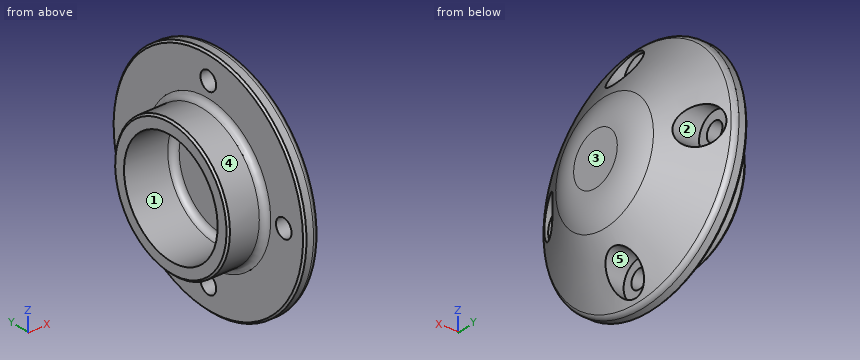
```python
from build123d import *

# Parameters (mm, degrees)
FILLET2_R          = 1
CHAMFER1_SIZE      = 0.3
SKETCH2_R          = 1.5
CUT_EXTRUDE1_DEPTH = 10
SKETCH3_R          = 3
CUT_EXTRUDE2_DEPTH = 10


with BuildPart() as part:
    # Sketch1 → Revolve1 (revolve)
    with BuildSketch(Plane.XY, mode=Mode.PRIVATE) as revolve1_sk:
        with BuildLine():
            Line((-6, 9), (-6, 11))
            Line((-6, 11), (0, 11))
            Line((0, 11), (0, 18.5))
            Line((0, 18.5), (1.438007651, 18.5))
            ThreePointArc((1.438007651, 18.5), (1.927932672, 18.371764575), (2.292206206, 18.019946947))
            Line((2.292206206, 18.019946947), (7.541985556, 9.395309443))
            ThreePointArc((7.541985556, 9.395309443), (8.628599471, 6.895853348), (9, 4.195839975))
            Line((9, 4.195839975), (9, 0))
            Line((9, 0), (2, 0))
            Line((2, 0), (2, 9))
            Line((2, 9), (-6, 9))
        make_face()
    revolve(revolve1_sk.sketch.rotate(Axis((0, 0, 0), (1, 0, 0)), 90), axis=Axis((0, 0, 0), (1, 0, 0)))

    # Fillet2
    fillet2_edges = [part.edges().sort_by_distance(p)[0] for p in [
        (0, 0, -11),
        (2, 0, -9),
    ]]
    fillet(fillet2_edges, radius=FILLET2_R)

    # Chamfer1
    chamfer1_edges = [part.edges().sort_by_distance(p)[0] for p in [
        (0, 0, -18.5),
        (-6, 0, -11),
    ]]
    chamfer(chamfer1_edges, length=CHAMFER1_SIZE)

    # Sketch2 → Cut-Extrude1 (cut)
    with BuildSketch(Plane.ZY):
        with Locations((0, 14.5)):
            Circle(SKETCH2_R)
        with Locations((14.5, 0)):
            Circle(SKETCH2_R)
        with Locations((0, -14.5)):
            Circle(SKETCH2_R)
        with Locations((-14.5, 0)):
            Circle(SKETCH2_R)
    extrude(amount=-CUT_EXTRUDE1_DEPTH, mode=Mode.SUBTRACT)

    # Sketch3 → Cut-Extrude2 (cut)
    with BuildSketch(Plane.ZY.offset(-2)):
        with Locations((0, 14.5)):
            Circle(SKETCH3_R)
        with Locations((14.5, 0)):
            Circle(SKETCH3_R)
        with Locations((0, -14.5)):
            Circle(SKETCH3_R)
        with Locations((-14.5, 0)):
            Circle(SKETCH3_R)
    extrude(amount=-CUT_EXTRUDE2_DEPTH, mode=Mode.SUBTRACT)


solid = part.part
```
Read the model definition and answer for the solid it produces. Units are mm, in the model's axes. Face numbers are marked on the shaded views. A direction names the side the tool comes from. Round coordinates to 2 decimals unless told otherwise and drop trailing zeros. Write each loop counter-clockwise with the first axis right and the second up, starting at its lowest first coordinate (ties: lowest second). Pieces come first, ordered by that corner, then holes. Notation, with made-up numbers: (86.5, 1) - (116.5, 1) arc R24 ccw to (116.5, 27) - close; hole circle Ø8 at (-33, 7). An arc over 180 degrees is marked (long way). Use CSV: the item, a comma, the result in double quotes.
Q1. Determine the mould class of the marked faces 3, 4 and 5 for opening direction Y: +Y half, -Y half, draft (parallel to the pull), parting line (faces both ways), or undercut.
Values:
face 3,"draft"
face 4,"parting line"
face 5,"undercut"
Q2. Find section D-D, the plane x = 7. Write down the section's boundary in (y, z).
Values:
outline,"circle Ø20.57 at (0, 0)"
Q3. Find section A-A, the plane y = 0. Count the separate pieces of the cut face and the enclosed holes in it, then the cut area to 3 significant figures.
Values:
separate pieces,"3"
enclosed holes,"0"
area,"198 mm²"
Q4. Find section B-B, the plane x = -1.5. Write down the section's boundary in (y, z), then the cut area to 3 significant figures.
Values:
outline,"circle Ø22 at (0, 0); hole circle Ø18 at (0, 0)"
area,"126 mm²"
Q5. Straight lines are drawn through the part: line 1 along Y through (x, z) = (0.9, 0); line 2 along Y through (x, z) = (-2.5, 0); line 3 along Y through (x, z) = (1.5, 6). For each, find the intervals that lie inside material, in ascending order.
Values:
line 1,"y = -18.5 to -16, -13 to -9, 9 to 13, 16 to 18.5"
line 2,"y = -11 to -9, 9 to 11"
line 3,"y = -17.5 to -6.53, 6.53 to 17.5"
Q6. A tool of negligible diameter and unlimited length cuts with its end or side. For the marked faces 1 and 2, from which of +Z, -Z, +X, -X, +Y, -Y can it reach the whole face along a straight path? Write none if from no direction.
Values:
face 1,"-X"
face 2,"+X"
Q7. Each of these flat-tipped pins is pushed along its axis until it touches: pin 1 Ø3.5 at (y, z) = (0, -14.5) entering from -X; pin 2 Ø5 at (x, y) = (1, 11) entering from -Z; pin 3 Ø1.8 at (y, z) = (0, 14.5) entering from +X; pin 4 Ø3.5 at (y, z) = (-14.5, 0) entering from +X. Where does it stop, or does it pass through?
Values:
pin 1,"stops at x = 0"
pin 2,"stops at z = -16.43"
pin 3,"passes through"
pin 4,"stops at x = 2"
